The listing builds one solid part. Answer for the finished solid, in the listing's coordinates (mm). A direction names the side the tool comes from. Coordinates: 2 decimals unless noted, no trailing zeros. Order: outer loops, then holes, each group sorted by start corner. A loop starts at its lowest first (then second) coordinate and runs counter-clockwise, first axis right, second up.
Autodesk Inventor part; units mm, degrees
ref_plane "YZ Plane" through (0, 0, 0) normal (1, 0, 0) x (0, 1, 0)
ref_plane "XZ Plane" through (0, 0, 0) normal (0, 1, 0) x (-1, 0, 0)
ref_plane "XY Plane" through (0, 0, 0) normal (0, 0, 1) x (1, 0, 0)
sketch "Sketch1" plane through (0, 0, 0) normal (0, 0, 1) x (1, 0, 0)
  line L0 (0, 133.1936) -> (0, -174.4071)
  line L1 (-87.3177, 0) -> (127.2932, 0)
  line L2 (8, -10.1) -> (-8, -10.1)
  line L3 (-8, -10.1) -> (-8, 10.1)
  line L4 (-8, 10.1) -> (8, 10.1)
  line L5 (8, 10.1) -> (8, -10.1)
  line L6 (8, -10.1) -> (-8, 10.1) construction
  line L7 (-8, -10.1) -> (8, 10.1) construction
  circle A0 centre (-6.731, 8.636) radius 0.5139 construction
  circle A1 centre (6.731, -8.763) radius 0.49 construction
  line L8 (-5.9376, -4.2616) -> (5.9143, -4.2616)
  line L9 (5.9143, -4.2616) -> (5.9143, -6.7235)
  line L10 (5.9143, -6.7235) -> (-5.9376, -6.7235)
  line L11 (-5.9376, -6.7235) -> (-5.9376, -4.2616)
  line L12 (-1.9876, 12.1457) -> (1.9674, 12.1457)
  line L13 (1.9674, 12.1457) -> (1.9674, 8.0874)
  line L14 (1.9674, 8.0874) -> (-1.9876, 8.0874)
  line L15 (-1.9876, 8.0874) -> (-1.9876, 12.1457)
  line L16 (-7.2449, 5.8703) -> (-1.7339, 5.8703)
  line L17 (-1.7339, 5.8703) -> (-1.7339, 0.8708)
  line L18 (-1.7339, 0.8708) -> (-7.2449, 0.8708)
  line L19 (-7.2449, 0.8708) -> (-7.2449, 5.8703)
  line L20 (-5.683, -0.4539) -> (-1.9876, -0.4539)
  line L21 (-1.9876, -0.4539) -> (-1.9876, -3.3033)
  line L22 (-1.9876, -3.3033) -> (-5.683, -3.3033)
  line L23 (-5.683, -3.3033) -> (-5.683, -0.4539)
  line L24 (-1.184, 4.5949) -> (6.731, 4.5949)
  line L25 (6.731, 4.5949) -> (6.731, -3.3033)
  line L26 (6.731, -3.3033) -> (-1.184, -3.3033)
  line L27 (-1.184, -3.3033) -> (-1.184, 4.5949)
  line L28 (54.8091, 13.2903) -> (96.6345, 13.2903) construction
  line L29 (96.6345, 13.2903) -> (96.6345, -86.1085) construction
  line L30 (96.6345, -86.1085) -> (54.8091, -86.1085) construction
  line L31 (54.8091, -86.1085) -> (54.8091, 13.2903) construction
  line L32 (-7.642, -75.3683) -> (-7.642, -85.3683)
  line L33 (71.1512, 85.7776) -> (64.977, -130.4641) construction
  line L34 (64.977, -130.4641) -> (-56.659, -126.9911) construction
  line L35 (-56.659, -126.9911) -> (-50.4848, 89.2506) construction
  line L36 (-50.4848, 89.2506) -> (71.1512, 85.7776) construction
  point P0 (0, 0)
  dimension "d0" = 16
  dimension "d54" = 20.2
  dimension "d67" = 8.636
  dimension "d68" = 6.731
  dimension "d69" = 8.763
  dimension "d70" = 6.731
  dimension "d173" = 17.399
  dimension "d175" = 10
  dimension "d232" = 13.462
extrude "Extrusion1" add sketch "Sketch1" against normal blind 1 contours L4 L13 L14 L0 | L0 L14 L15 L4 | L14 L13 L4 L5 L1 L25 L24 L0 | L0 L24 L27 L1 L3 L4 L15 L14 | L24 L25 L1 L0 | L0 L1 L27 L24 | L1 L25 L26 L0 | L0 L26 L27 L1 | L1 L27 L26 L0 L8 L11 L10 L2 L3 | L5 L2 L0 L10 L9 L8 L26 L25 L1 | L8 L9 L10 L0 | L0 L10 L11 L8 | L16 L17 L18 L19 | L20 L21 L22 L23
extrude "Extrusion2" add sketch "Sketch1" along normal blind 1 contours L24 L25 L1 L0 | L0 L1 L27 L24 | L1 L25 L26 L0 | L0 L26 L27 L1 | L16 L17 L18 L19 | L20 L21 L22 L23
extrude "Extrusion3" add sketch "Sketch1" along normal blind 1.5 contours L12 L13 L4 L0 | L0 L4 L15 L12 | L4 L13 L14 L0 | L0 L14 L15 L4 | L8 L9 L10 L0 | L0 L10 L11 L8
hole "Hole1" at (6.731, -8.763, 0) at (-6.731, 8.636, 0) direction (0, 0, -1) diameter 1 depth 25.4 tip angle 118
(1) Find section D-D (x = 0.5). Write down the section's boundary in (y, z).
(2) Find section C-C (y = 2). Write down the section's boundary in (x, z).
(3) The mould has two halves that part along Y. Classify faces 1 (the face through (-7.245, 3.3, 0.5)), 2 (the face through (2.8, -3.303, 0.5)): released by +Y, released by -Y, zero draft, split by the parting line, or undercut.
(4) Each of these flat-tipped pins is pushed along its axis until it touches: pin 1 Ø0.5 at (x, z) = (-4, 0.5) entering from -Y; pin 2 Ø0.5 at (y, z) = (2.5, 0.5) entering from -X; pin 3 Ø3 at (x, y) = (-4, -2.5) entering from +Z. Where does it stop, or does it pass through?
(5) Find section A-A (z = 0.35). Write down the section's boundary in (x, y), and give its area (3 significant figures).
(6) For faces 3 (the face through (0, 8.087, 1)), 4 (the face through (0, 11, 0)), 5 (the face through (6.731, 0.7, 0.5)), 6 (the face through (1.967, 10, 1)), 7 (the face through (-1.734, 3.4, 0.5)), determine the directions among +Z, -Z, +X, -X, +Y, -Y from which every point of the face is accessible in a straight line to the end or side of a thin tool.
(7) Consider line 1 (Y direction, x = -1, z = 0.4); line 2 (Y direction, x = 6.75, z = -0.8); line 3 (Y direction, x = -0.25, z = 1.05). Determine where each line is inside the solid, lowest interval first.
(8) Find section B-B (x = -3.25). Write down the section's boundary in (y, z).
Findings below:
1. outline: (-10.1, -1) - (10.1, -1) - (10.1, 0) - (12.15, 0) - (12.15, 1.5) - (8.09, 1.5) - (8.09, 0) - (4.59, 0) - (4.59, 1) - (-3.3, 1) - (-3.3, 0) - (-4.26, 0) - (-4.26, 1.5) - (-6.72, 1.5) - (-6.72, 0) - (-10.1, 0) - close
2. outline: (-8, -1) - (8, -1) - (8, 0) - (6.73, 0) - (6.73, 1) - (-1.18, 1) - (-1.18, 0) - (-1.73, 0) - (-1.73, 1) - (-7.24, 1) - (-7.24, 0) - (-8, 0) - close
3. face 1: zero draft
3. face 2: undercut
4. pin 1: stops at y = -6.72
4. pin 2: stops at x = -7.24
4. pin 3: stops at z = 1
5. outline: (-7.24, 0.87) - (-1.73, 0.87) - (-1.73, 5.87) - (-7.24, 5.87) - close; (-5.94, -6.72) - (5.91, -6.72) - (5.91, -4.26) - (-5.94, -4.26) - close; (-5.68, -3.3) - (-1.99, -3.3) - (-1.99, -0.45) - (-5.68, -0.45) - close; (-1.99, 8.09) - (1.97, 8.09) - (1.97, 12.15) - (-1.99, 12.15) - close; (-1.18, -3.3) - (6.73, -3.3) - (6.73, 4.59) - (-1.18, 4.59) - close
5. area: 146 mm2
6. face 3: +Z, +X, -X
6. face 4: -Z, +X, -X, +Y
6. face 5: +Z, +X, +Y, -Y
6. face 6: +Z, +X, +Y
6. face 7: +Z
7. line 1: y = -6.72 to -4.26, -3.3 to 4.59, 8.09 to 12.15
7. line 2: y = -10.1 to -9.26, -8.26 to 10.1
7. line 3: y = -6.72 to -4.26, 8.09 to 12.15
8. outline: (-10.1, -1) - (10.1, -1) - (10.1, 0) - (5.87, 0) - (5.87, 1) - (0.87, 1) - (0.87, 0) - (-0.45, 0) - (-0.45, 1) - (-3.3, 1) - (-3.3, 0) - (-4.26, 0) - (-4.26, 1.5) - (-6.72, 1.5) - (-6.72, 0) - (-10.1, 0) - close
